Check sheet for the drawn part. Datum: minimum x, y, z corner. Units: mm. A direction names the side the tool comes from. Coordinates: 2 decimals unless noted, no trailing zeros. Order: outer loops, then holes, each group sorted by start corner. A loop starts at its lowest first (then second) coordinate and runs counter-clockwise, first axis right, second up. Notation, with made-up numbers: M 13,81.5 L 69,81.5 A20 cw 69,116.5 Z; hole C 46,-6 d10. An arc over 180 degrees is marked long. Answer in a Markdown table with one row per item. Add a question column.
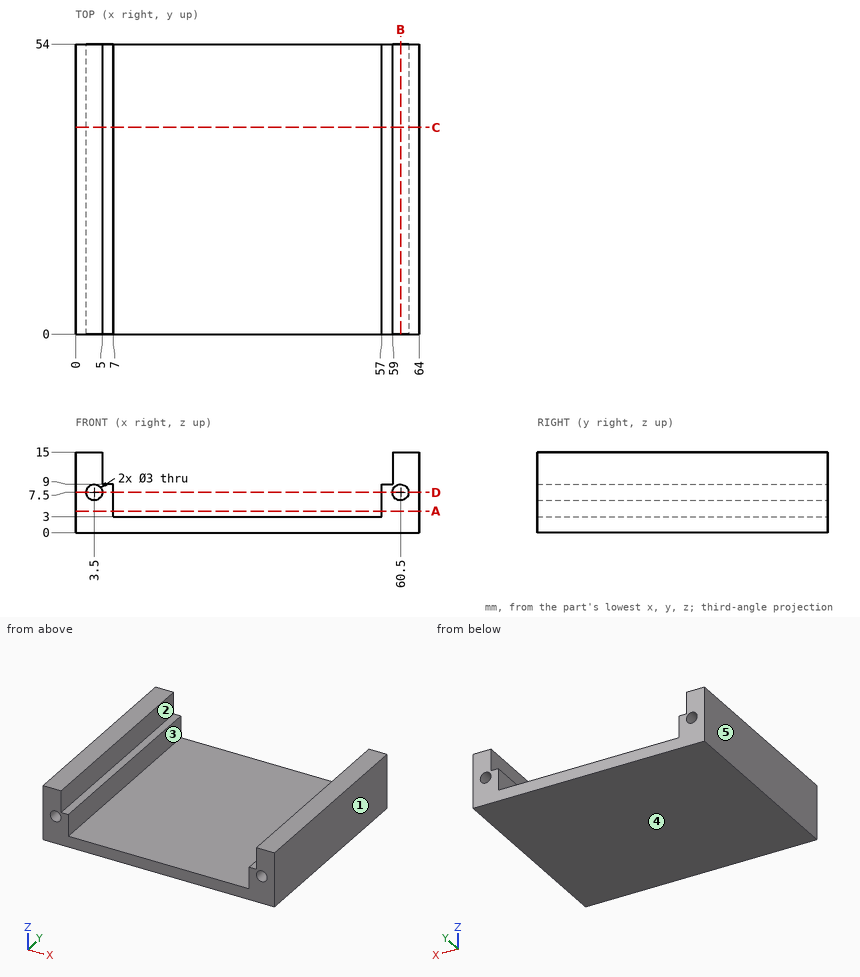
1. Set-up check for the marked faces 1 and 2: record each of +Z, -Z, +X, -X, +Y, -Y from which the full face is reachable in a straight line by a thin tool's end or side.
2. Scan lines: line 1 (X direction, y = 18, z = 7.5); line 2 (Z direction, x = 3.5, y = 32.5); line 3 (X direction, y = 23.5, z = 5). Record each from-to range of solid material in increasing order.
3. Section check B-B on x = 60.5. Enter the section's corners in (y, z).
4. Section check C-C on y = 38.5. Enter the section's corners in (x, z), then the cut area to 3 significant figures.
5. Section check A-A on z = 4. Enter the section's corners in (x, y).
6. Go/stop test with flat-tipped pins: pin 1 Ø5 at (x, y) = (18.5, 39) entering from +Z; pin 2 Ø1.8 at (x, z) = (60.5, 7.5) entering from +Y; pin 3 Ø1.6 at (x, y) = (57.5, 32) entering from +Z. Record where each tip stops, or that it passes through.
7. Section check D-D on z = 7.5. Enter the section's corners in (x, y).
8. Release check for a two-part mould opening along X. For the marked faces 3, 4 and 5 record: released by +X, released by -X, zero draft, split by the parting line, or undercut.
Result sheet:
| question | item | result |
|---|---|---|
| 1 | face 1 | +Z, -Z, +X, +Y, -Y |
| 1 | face 2 | +Z, +Y, -Y |
| 2 | line 1 | 0 to 2, 5 to 7, 57 to 59, 62 to 64 |
| 2 | line 2 | 0 to 6, 9 to 15 |
| 2 | line 3 | 0 to 7, 57 to 64 |
| 3 | outline | M 0,0 L 54,0 L 54,6 L 0,6 Z; M 0,9 L 54,9 L 54,15 L 0,15 Z |
| 4 | outline | M 0,0 L 64,0 L 64,15 L 59,15 L 59,9 L 57,9 L 57,3 L 7,3 L 7,9 L 5,9 L 5,15 L 0,15 Z; hole C 3.5,7.5 d3; hole C 60.5,7.5 d3 |
| 4 | area | 322 mm^2 |
| 5 | outline | M 0,0 L 7,0 L 7,54 L 0,54 Z; M 57,0 L 64,0 L 64,54 L 57,54 Z |
| 6 | pin 1 | z = 3 |
| 6 | pin 2 | through |
| 6 | pin 3 | z = 9 |
| 7 | outline | M 0,0 L 2,0 L 2,54 L 0,54 Z; M 5,0 L 7,0 L 7,54 L 5,54 Z; M 57,0 L 59,0 L 59,54 L 57,54 Z; M 62,0 L 64,0 L 64,54 L 62,54 Z |
| 8 | face 3 | undercut |
| 8 | face 4 | zero draft |
| 8 | face 5 | released by -X |
